```python
from build123d import *

# Parameters (mm, degrees)
BOSS_EXTRUDE1_DEPTH = 43
CUT_EXTRUDE1_START  = -8.55
SKETCH3_W           = 66.07
SKETCH3_H           = 38
CUT_EXTRUDE1_DEPTH  = 8.55
SKETCH4_W           = 47.5
SKETCH4_H           = 37
CUT_EXTRUDE2_DEPTH  = 0.6
CUT_EXTRUDE3_REACH  = 57.993
SKETCH5_W           = 38.5
SKETCH5_H           = 35.2
FILLET1_R           = 7
FILLET2_R           = 10
SKETCH6_W           = 0.5
SKETCH6_H           = 38
CUT_EXTRUDE4_DEPTH  = 10
SKETCH7_W           = 14.712909767
SKETCH7_H           = 38
BOSS_EXTRUDE2_DEPTH = 1.5
CUT_EXTRUDE5_REACH  = 57.044
SKETCH8_W           = 14.712909767
SKETCH8_H           = 38
SKETCH9_W           = 15
SKETCH9_H           = 38
BOSS_EXTRUDE3_DEPTH = 3


with BuildPart() as part:
    # Sketch1 → Boss-Extrude1 (new body)
    with BuildSketch(Plane.XY.offset(21.5)):
        with BuildLine():
            Line((21.074737692, 0), (21.074737692, 9.75))
            Line((21.074737692, 9.75), (-49.995262308, 9.75))
            Line((-49.995262308, 9.75), (-49.995262308, -3.418305859))
            ThreePointArc((-49.995262308, -3.418305859), (-41.302219327, -0.862388361), (-32.282352541, 0))
            Line((-32.282352541, 0), (21.074737692, 0))
        make_face()
    extrude(amount=-BOSS_EXTRUDE1_DEPTH)

    # Sketch3 → Cut-Extrude1 (cut)
    with BuildSketch(Plane(origin=(0, 8.55, 0), x_dir=(1, 0, 0), z_dir=(0, 1, 0)).offset(CUT_EXTRUDE1_START)):
        with Locations((-14.460262308, 0)):
            Rectangle(SKETCH3_W, SKETCH3_H)
    extrude(amount=CUT_EXTRUDE1_DEPTH, mode=Mode.SUBTRACT)

    # Sketch4 → Cut-Extrude2 (cut)
    with BuildSketch(Plane.XZ.offset(-8.55)):
        with Locations((-14.460262308, 0)):
            Rectangle(SKETCH4_W, SKETCH4_H)
    extrude(amount=-CUT_EXTRUDE2_DEPTH, mode=Mode.SUBTRACT)

    # Sketch5 → Cut-Extrude3 (cut, up to next)
    with BuildSketch(Plane(origin=(0, 9.75, 0), x_dir=(-1, 0, 0), z_dir=(0, 1, 0)), mode=Mode.PRIVATE) as cut_extrude3_sk1:
        with Locations((10.460262308, 0)):
            Rectangle(SKETCH5_W, SKETCH5_H)
    cut_extrude3_tool1 = extrude(cut_extrude3_sk1.sketch, amount=-CUT_EXTRUDE3_REACH, mode=Mode.PRIVATE) & part.part
    add(cut_extrude3_tool1.solids().sort_by_distance((-10.460262, 9.75, 0))[0], mode=Mode.SUBTRACT)

    # Fillet1
    fillet1_edges = [part.edges().sort_by_distance(p)[0] for p in [
        (18.574737692, 8.55, 0),
        (-47.495262308, 8.55, 0),
    ]]
    fillet(fillet1_edges, radius=FILLET1_R)

    # Fillet2
    # the kernel refuses this fillet: 10 mm, written as the material it takes off along each edge
    with BuildSketch(Plane(origin=(21.074737692, 9.75, 46.492186279), x_dir=(0, -1, 0), z_dir=(0, 0, -1))) as fillet2_piece_1:
        with BuildLine():
            CenterArc((10, 9.996874512), FILLET2_R, 180, 88.567456262)
            Line((0, 9.996874512), (-0.2, 9.996874512))
            Line((-0.2, 9.996874512), (-0.2, 0))
            Line((-0.2, 0), (0, -0.2))
            ThreePointArc((0, -0.2), (4.875, -0.2), (9.745, -0.19993749))
            Line((9.745, -0.19993749), (9.75, 0))
        make_face()
    extrude(amount=92.984372558, mode=Mode.SUBTRACT)
    with BuildSketch(Plane(origin=(-49.995262308, 9.75, 46.5), x_dir=(1, 0, 0), z_dir=(0, 0, -1))) as fillet2_piece_2:
        with BuildLine():
            CenterArc((FILLET2_R, FILLET2_R), FILLET2_R, 180, 90)
            Line((0, FILLET2_R), (-FILLET2_R * 0.02, FILLET2_R))
            Line((-FILLET2_R * 0.02, FILLET2_R), (-FILLET2_R * 0.02, -FILLET2_R * 0.02))
            Line((-FILLET2_R * 0.02, -FILLET2_R * 0.02), (FILLET2_R, -FILLET2_R * 0.02))
            Line((FILLET2_R, -FILLET2_R * 0.02), (FILLET2_R, 0))
        make_face()
    extrude(amount=93, mode=Mode.SUBTRACT)

    # Sketch6 → Cut-Extrude4 (cut)
    with BuildSketch(Plane(origin=(0, 0, 0), x_dir=(1, 0, 0), z_dir=(0, 1, 0))):
        with Locations((-32.532352541, 0)):
            Rectangle(SKETCH6_W, SKETCH6_H)
    extrude(amount=-CUT_EXTRUDE4_DEPTH, mode=Mode.SUBTRACT)

    # Sketch7 → Boss-Extrude2 (add)
    with BuildSketch(Plane(origin=(0, 0, 0), x_dir=(1, 0, 0), z_dir=(0, 1, 0))):
        with Locations((-40.138807425, 0)):
            Rectangle(SKETCH7_W, SKETCH7_H)
    extrude(amount=BOSS_EXTRUDE2_DEPTH)

    # Sketch8 → Cut-Extrude5 (cut, up to next)
    with BuildSketch(Plane(origin=(0, 1.5, 0), x_dir=(1, 0, 0), z_dir=(0, 1, 0)), mode=Mode.PRIVATE) as cut_extrude5_sk1:
        with Locations((-40.138807425, 0)):
            Rectangle(SKETCH8_W, SKETCH8_H)
    cut_extrude5_tool1 = extrude(cut_extrude5_sk1.sketch, amount=-CUT_EXTRUDE5_REACH, mode=Mode.PRIVATE) & part.part
    add(cut_extrude5_tool1.solids().sort_by_distance((-40.138807, 1.5, 0))[0], mode=Mode.SUBTRACT)

    # Sketch9 → Boss-Extrude3 (add)
    with BuildSketch(Plane.XZ):
        with Locations((11.074737692, 0)):
            Rectangle(SKETCH9_W, SKETCH9_H)
    extrude(amount=-BOSS_EXTRUDE3_DEPTH)


solid = part.part
```
The model under review builds one solid part; all positions refer to its coordinate system, in mm. A direction names the side the tool comes from. Coordinates: 2 decimals unless noted, no trailing zeros. Loops run counter-clockwise (first coordinate to the right, second up) from the corner with the lowest first, then second, coordinate; pieces in that order, holes last. Notation, with made-up numbers: (50.25, 40) -> (81.25, 40) arc R26 ccw to (81.25, 73) -> close; hole circle Ø4 at (3, 57.5). An arc over 180 degrees is marked (long way). Answer as CSV lines item,"result".
Item 1: Take a section at B-B, the plane z = -2. State the section outline as (x, y) points.
Results below:
outline,"(-50, -3.42) arc R47.6 cw to (-47.5, -2.5) -> (-47.5, 1.55) arc R7 cw to (-40.5, 8.55) -> (-38.21, 8.55) -> (-38.21, 9.15) -> (-29.71, 9.15) -> (-29.71, 9.75) -> (-40, 9.75) arc R10 ccw to (-50, -0.25) -> close; (3.57, 0) -> (21.07, 0) arc R10 ccw to (11.08, 9.75) -> (8.79, 9.75) -> (8.79, 9.15) -> (9.29, 9.15) -> (9.29, 8.55) -> (11.57, 8.55) arc R7 cw to (18.42, 3) -> (3.57, 3) -> close"
Item 2: Take a section at D-D, the plane y = 6. State the section outline as (x, z) points.
Results below:
outline,"(-47.8, -21.5) -> (18.88, -21.5) -> (18.88, 21.5) -> (-47.8, 21.5) -> close; hole (-45.9, -19) -> (16.98, -19) -> (16.98, 19) -> (-45.9, 19) -> close"
Item 3: Draft analysis for pull direction X (two halves, no side actions). For faces 5 (the flat face through (-15, 4, -19)), 6 (the flat face through (-49.995, -2, 0)), 7 (the flat face through (-15, 5, -21.5)), 8 (the cylindrical face through (17.982, 6.984, 0.301)), state which applies: +X half, -X half, draft (parallel to the pull), parting line (faces both ways), or undercut.
Results below:
face 5,"undercut"
face 6,"-X half"
face 7,"draft"
face 8,"+X half"
Item 4: Take a section at A-A, the plane x = -13. State the section outline as (y, z) points.
Results below:
outline,"(0, -21.5) -> (9.75, -21.5) -> (9.75, -17.6) -> (9.15, -17.6) -> (9.15, -18.5) -> (8.55, -18.5) -> (8.55, -19) -> (0, -19) -> close; (0, 19) -> (8.55, 19) -> (8.55, 18.5) -> (9.15, 18.5) -> (9.15, 17.6) -> (9.75, 17.6) -> (9.75, 21.5) -> (0, 21.5) -> close"
Item 5: Machinability: for faces 1 (the cylindrical face through (-45.499, 6.445, -0.266)), 2 (the flat face through (-15, 5, 21.5)), 3 (the cylindrical face through (16.03, 6.95, -0.27)), 4 (the flat face through (6, 0, 5)), which of the approach directions +Z, -Z, +X, -X, +Y, -Y give a long, thin tool a straight path to every point of the face, cutting with its end or side? Answer none if there is none.
Results below:
face 1,"-Y"
face 2,"+Z, +X, -X, +Y, -Y"
face 3,"none"
face 4,"+Z, -Z, +X, -Y"
Item 6: For L1, parallel to Z at x = -15.5, y = 2.75; L2, parallel to Y at x = -33, z = -5; L3, parallel to X at y = 2.75, z = 5, list the stretches that pass through material, from the lowest coordinate up.
Results below:
L1,"z = -21.5 to -19, 19 to 21.5"
L2,"y = 9.15 to 9.75"
L3,"x = -49.53 to -47.39, 3.57 to 20.62"
Item 7: Take a section at C-C, the plane x = 5. State the section outline as (y, z) points, and give its area (3 significant figures).
Results below:
outline,"(0, -21.5) -> (9.75, -21.5) -> (9.75, -17.6) -> (9.15, -17.6) -> (9.15, -18.5) -> (8.55, -18.5) -> (8.55, -19) -> (3, -19) -> (3, 19) -> (8.55, 19) -> (8.55, 18.5) -> (9.15, 18.5) -> (9.15, 17.6) -> (9.75, 17.6) -> (9.75, 21.5) -> (0, 21.5) -> close"
area,"165 mm2"
Item 8: Insertion check: pin 1 (1 mm diameter, centred on x = 11, z = -1.5, fed in from -Y); pin 2 (0.7 mm diameter, centred on y = 9, z = -7, fed in from -X); pin 3 (2 mm diameter, centred on y = -1.5, z = 3.5, fed in from +X). Each pin has a flat end and moves straight along its axis. Give the tip position at first contact, or say it passes through.
Results below:
pin 1,"stops at y = 0"
pin 2,"stops at x = -44.55"
pin 3,"stops at x = -47.5"
